Autodesk Inventor part; units mm, degrees
ref_plane "Work Plane1" through (0, -20, 50) normal (0, 0, -1) x (-1, 0, 0)
ref_plane "YZ Plane" through (0, 0, 0) normal (1, 0, 0) x (0, 1, 0)
ref_plane "XZ Plane" through (0, 0, 0) normal (0, 1, 0) x (-1, 0, 0)
sketch "Sketch2" plane through (0, 0, 0) normal (0, 0, 1) x (1, 0, 0)
  line L0 (-20, 20) -> (20, 20)
  line L1 (20, 20) -> (20, -20)
  line L2 (20, -20) -> (-20, -20)
  line L3 (-20, -20) -> (-20, 20)
  line L4 (-20, 20) -> (20, -20) construction
  line L5 (20, 20) -> (-20, -20) construction
  point P0 (0, 0)
  dimension "d5" = 40
  dimension "d6" = 40
extrude "Extrusion2" add sketch "Sketch2" along normal blind 50
sketch "Sketch3" plane through (20, -20, 0) normal (1, 0, 0) x (0, 0, -1)
  line L0 (0, 40) -> (-50, 40)
  line L1 (0, 0) -> (-50, 0)
  line L2 (0, 40) -> (-10, 40)
  line L3 (-10, 40) -> (-10, 0)
  line L4 (-10, 0) -> (0, 0)
  line L5 (0, 0) -> (0, 40)
  point P0 (0, 20)
  dimension "d9" = 10
extrude "Extrusion3" add sketch "Sketch3" along normal blind 40
sketch "Sketch4" plane through (-20, -20, 0) normal (-1, 0, 0) x (0, 0, 1)
  line L0 (0, 40) -> (0, 0)
  line L1 (0, 40) -> (50, 40)
  line L2 (0, 0) -> (10, 0)
  line L3 (10, 0) -> (10, 40)
  line L4 (10, 40) -> (0, 40)
  line L5 (0, 40) -> (0, 0)
  point P0 (0, 20)
  dimension "d13" = 10
extrude "Extrusion4" add sketch "Sketch4" along normal blind 40
sketch "Sketch5" plane through (-20, -20, 10) normal (0, 0, 1) x (1, 0, 0)
  line L0 (0, 40) -> (0, 0)
  line L1 (-40, 0) -> (80, 0)
  line L2 (-20, 40) -> (-40, 40)
  line L3 (-40, 40) -> (-40, 0)
  line L4 (-40, 0) -> (-20, 0)
  line L5 (0, 0) -> (0, 40)
  circle A0 centre (-20, 20) radius 10
  arc A1 (-20, 40) -> (-20, 0) centre (-20, 20) ccw
  line L6 (0, 40) -> (-40, 40)
  line L7 (0, 0) -> (-40, 0)
  line L8 (-40, 0) -> (-40, 40)
  line L9 (60, 0) -> (80, 0)
  line L10 (80, 0) -> (80, 40)
  line L11 (80, 40) -> (60, 40)
  circle A2 centre (60, 20) radius 10
  arc A3 (60, 0) -> (60, 40) centre (60, 20) ccw
  line L12 (40, 40) -> (80, 40)
  line L13 (80, 40) -> (80, 0)
  line L14 (40, 0) -> (80, 0)
  point P0 (20, 20)
  point P1 (80, 20)
  point P2 (-40, 20)
extrude "Extrusion5" cut sketch "Sketch5" against normal through all contours A3 L11 L10 | A3 L10 L1 | A1 L3 L2 | L1 L3 A1 | A0 | A2
sketch "Sketch6" plane through (-20, -20, 50) normal (0, -1, 0) x (1, 0, 0)
  line L0 (0, -40) -> (-20, -40)
  line L1 (40, -40) -> (40, 0)
  line L2 (40, -20) -> (40, 0)
  line L3 (40, 0) -> (0, 0)
  line L4 (0, 0) -> (0, -20)
  arc A0 (40, -20) -> (0, -20) centre (20, -20) ccw
  circle A1 centre (20, -20) radius 10
  line L5 (0, 0) -> (40, 0)
  line L6 (40, -40) -> (40, 0)
  line L7 (0, -40) -> (0, 0)
  point P0 (20, -50)
  point P1 (20, 0)
  dimension "d20" = 20
extrude "Extrusion6" cut sketch "Sketch6" against normal through all
ref_plane "Work Plane1" through (0, -20, 50) normal (0, 0, -1) x (-1, 0, 0)
sketch "Sketch8" plane through (0, -20, 50) normal (0, 0, -1) x (-1, 0, 0)
  circle A0 centre (0, 20) radius 2.5
  dimension "d31" = 5
extrude "Extrusion7" cut sketch "Sketch8" along normal blind 12
thread "Thread1"
thread "Thread2"
thread "Thread3"
properties part number "06022024_ejercicio"
The model under review builds one solid part; all positions refer to its coordinate system, in mm. A direction names the side the tool comes from. Round coordinates to 2 decimals unless told otherwise and drop trailing zeros. Loops run counter-clockwise (first coordinate to the right, second up) from the corner with the lowest first, then second, coordinate; pieces in that order, holes last. Notation, with made-up numbers: M -14,51 L 22,51 A17 ccw 22,59 Z; hole C 3.25,-33.5 d10. An arc over 180 degrees is marked long. Put each result on its own line as item: value.
Q1. Machinability: for faces 1 (the cylindrical face through (-2.385, -0.751, 44.913)), 2 (the flat face through (-20, 0, 20)), 3 (the flat face through (20, 0, 20)), which of the approach directions +Z, -Z, +X, -X, +Y, -Y give a long, thin tool a straight path to every point of the face, cutting with its end or side? Answer none if there is none.
Result set:
face 1: +Z
face 2: +Z, -X, +Y, -Y
face 3: +Z, +X, +Y, -Y
Q2. Mouldability with a two-part tool opening along Z and no side actions: class faces 4 (the flat face through (-31, -5, 10)), 5 (the flat face through (1, -20, 19)), 6 (the cylindrical face through (-2.17, -0.28, 20.24)), 7 (the flat face through (1, 0, 0)) as released by +Z, released by -Z, zero draft, split by the parting line, or undercut.
Result set:
face 4: released by +Z
face 5: zero draft
face 6: undercut
face 7: released by -Z
Q3. Consider section A-A, the plane y = -8.5. Give the boundary of the cut face in (x, z).
Result set:
outline: M -58.1,0 L -45.27,0 L -45.27,10 L -58.1,10 Z; M -34.73,0 L 34.73,0 L 34.73,10 L 20,10 L 20,30 A20 ccw -20,30 L -20,10 L -34.73,10 Z; M 45.27,0 L 58.1,0 L 58.1,10 L 45.27,10 Z; hole C 0,30 d20
Q4. Consider section D-D, the plane y = 0. Give the boundary of the cut face in (x, z).
Result set:
outline: M -60,0 L -50,0 L -50,10 L -60,10 Z; M -30,0 L 30,0 L 30,10 L 20,10 L 20,30 A20 ccw 2.5,49.84 L 2.5,39.68 A10 cw long -2.5,39.68 L -2.5,49.84 A20 ccw -20,30 L -20,10 L -30,10 Z; M 50,0 L 60,0 L 60,10 L 50,10 Z
Q5. For pin 1 (6 mm diameter, centred on y = 4.5, z = 15.5, fed in from -X); pin 2 (18 mm diameter, centred on x = 40, y = 0, fed in from -Z); pin 3 (12 mm diameter, centred on x = -30, y = -2.5, fed in from +Z); pin 4 (8 mm diameter, centred on y = 14.5, z = 38, fed in from +X), all flat-tipped, find the tip position at first contact; note any pin that passes through.
Result set:
pin 1: stops at x = -20
pin 2: passes through
pin 3: stops at z = 10
pin 4: stops at x = 19.6
Q6. To check wall thickness, follow L1, parallel to Y at x = -40, z = 3; L2, parallel to Y at x = 0, z = 42; L3, parallel to Z at x = 0, y = -1.5. State the ranges of each line that lie inside material, in increasing order.
Result set:
L1: y = -20 to -10, 10 to 20
L2: y = -20 to -2.5, 2.5 to 20
L3: z = 0 to 20
Q7. Consider section C-C, the plane z = 36.5. Give the boundary of the cut face in (x, y).
Result set:
outline: M -18.91,-20 L -7.6,-20 L -7.6,20 L -18.91,20 Z; M 7.6,-20 L 18.91,-20 L 18.91,20 L 7.6,20 Z
Q8. Consider section B-B, the plane x = 0. Give the boundary of the cut face in (y, z), then the cut area to 3 significant figures.
Result set:
outline: M -20,0 L 20,0 L 20,20 L -20,20 Z; M -20,40 L -2.5,40 L -2.5,50 L -20,50 Z; M 2.5,40 L 20,40 L 20,50 L 2.5,50 Z
area: 1,150 mm²
